CAD build for the part. Positions are in the model's coordinates, mm. A direction names the side the tool comes from. Coordinates: 2 decimals unless noted, no trailing zeros. Loops run counter-clockwise (first coordinate to the right, second up) from the corner with the lowest first, then second, coordinate; pieces in that order, holes last. Notation, with made-up numbers: M 64,15 L 117,15 A20 ccw 117,33 Z; hole C 51,-39 d2. An arc over 180 degrees is marked long. Answer as a JSON object with one key per item and string values. Group by question number.
```python
from build123d import *

# Parameters (mm, degrees)
F1_DEPTH = 9.5
F2_W     = 9.5
F2_H     = 119.5
F2_H_2   = 9.5
F2_W_2   = 93
F3_DEPTH = 48
F5_DEPTH = 25.4


with BuildPart() as f1:
    # F0 (on Top) → F1 (new body)
    with BuildSketch(Plane.XY):
        Polygon((0, 129), (0, 0), (556, 0), (556, 43), (438, 43), (438, 114.0399202704), (426, 114.0399202704), (426, 33.5), (310, 33.5), (310, 83.1064879894), (302.5, 83.1064879894), (302.5, 129), align=None)
    extrude(amount=F1_DEPTH)

    # F2 (on face) → F3 (join)
    with BuildSketch(Plane.XY.offset(9.5)):
        with Locations((4.75, 69.25)):
            Rectangle(F2_W, F2_H)
        with Locations((4.75, 4.75)):
            Rectangle(F2_W, F2_H_2)
        with Locations((56, 4.75)):
            Rectangle(F2_W_2, F2_H_2)
        with Locations((107.25, 69.25)):
            Rectangle(F2_W, F2_H)
        with Locations((107.25, 4.75)):
            Rectangle(F2_W, F2_H_2)
    extrude(amount=F3_DEPTH)

    # F4 (on face) → F5 (cut)
    with BuildSketch(Plane.XY.offset(9.5)):
        with BuildLine():
            ThreePointArc((149.5, 64.5), (147, 67), (144.5, 64.5))
            Line((144.5, 64.5), (149.5, 64.5))
        make_face()
        with BuildLine():
            Line((149.5, 64.5), (144.5, 64.5))
            ThreePointArc((144.5, 64.5), (147, 62), (149.5, 64.5))
        make_face()
        with BuildLine():
            Line((283.5, 64.5), (278.5, 64.5))
            ThreePointArc((278.5, 64.5), (281, 62), (283.5, 64.5))
        make_face()
        with BuildLine():
            ThreePointArc((283.5, 64.5), (281, 67), (278.5, 64.5))
            Line((278.5, 64.5), (283.5, 64.5))
        make_face()
    extrude(amount=-F5_DEPTH, mode=Mode.SUBTRACT)


solid = f1.part
```
Item 1: Slice it at D-D, the plane x = 182. Write the cut outline in (y, z), then the cut area to 3 significant figures.
Item 2: Slice it at A-A, the plane y = 51.5. Write the cut outline in (x, z), then the cut area to 3 significant figures.
Item 3: Slice it at B-B, the plane z = 52.5. Write the cut outline in (x, y).
Item 4: Pin check, flat tips, straight feed: pin 1 (10.5 mm diameter, centred on y = 70, z = 4.5, fed in from +X); pin 2 (4 mm diameter, centred on x = 147, y = 64.5, fed in from -Z); pin 3 (2 mm diameter, centred on x = 475, y = 26, fed in from +Z); pin 4 (4 mm diameter, centred on y = 84.5, z = 36, fed in from +X). Stop position of each tip, or through.
Item 5: Slice it at C-C, the plane x = 96. Write the cut outline in (y, z), then the cut area to 3 significant figures.
Item 6: Tool access for faces 1 (the flat face through (432, 114.04, 5)), 2 (the flat face through (282, 51, 9.5)), 3 (the flat face through (102.5, 68, 33)), 4 (the flat face through (426, 74, 5)): list every direction of +Z, -Z, +X, -X, +Y, -Y with a clear straight run to the whole face (end or side of a thin tool).
Item 7: Drill centre lines: L1, parallel to X at y = 64, z = 3; L2, parallel to X at y = 123, z = 48; L3, parallel to Y at x = 147, z = 3.75. Where is each one in solid material? Low to high. Write a range as from..to.
Item 8: Pull direction X, two halves, no side cores. Call faces 5 (the flat face through (556, 21, 5)), 6 (the flat face through (369, 33.5, 5)), 7 (the flat face through (56, 7, 57.5)): released by +X, released by -X, zero draft, split by the parting line, or undercut.
Computed:
{
 "1": {"outline": "M 0,0 L 129,0 L 129,9.5 L 0,9.5 Z", "area": "1,230 mm2"},
 "2": {"outline": "M 0,0 L 310,0 L 310,9.5 L 112,9.5 L 112,57.5 L 102.5,57.5 L 102.5,9.5 L 9.5,9.5 L 9.5,57.5 L 0,57.5 Z; M 426,0 L 438,0 L 438,9.5 L 426,9.5 Z", "area": "3,970 mm2"},
 "3": {"outline": "M 0,0 L 112,0 L 112,129 L 102.5,129 L 102.5,9.5 L 9.5,9.5 L 9.5,129 L 0,129 Z"},
 "4": {"pin 1": "x = 438", "pin 2": "through", "pin 3": "z = 9.5", "pin 4": "x = 112"},
 "5": {"outline": "M 0,0 L 129,0 L 129,9.5 L 9.5,9.5 L 9.5,57.5 L 0,57.5 Z", "area": "1,680 mm2"},
 "6": {"face 1": "+Z, -Z, +X, +Y", "face 2": "+Z, +X, +Y, -Y", "face 3": "+Z, +Y", "face 4": "+Z, -Z, +Y"},
 "7": {"L1": "0..144.55, 149.45..278.55, 283.45..310, 426..438", "L2": "0..9.5, 102.5..112", "L3": "0..62, 67..129"},
 "8": {"face 5": "released by +X", "face 6": "undercut", "face 7": "zero draft"}
}
